Geometry: final body of the model. Coordinates: model frame, mm. Face numbers are marked on the shaded views. A direction names the side the tool comes from. Give positions to 0.01 mm unless a question says otherwise; leave off trailing zeros. Write each loop counter-clockwise with the first axis right and the second up, starting at its lowest first coordinate (ties: lowest second). Pieces come first, ordered by that corner, then holes. Notation, with made-up numbers: (12.25, 44) - (53.25, 44) arc R14 ccw to (53.25, 54) - close; hole circle Ø6 at (-28.5, -35.5). An arc over 180 degrees is marked (long way). One line per question, with ' | ' between items. Start each with the question number.
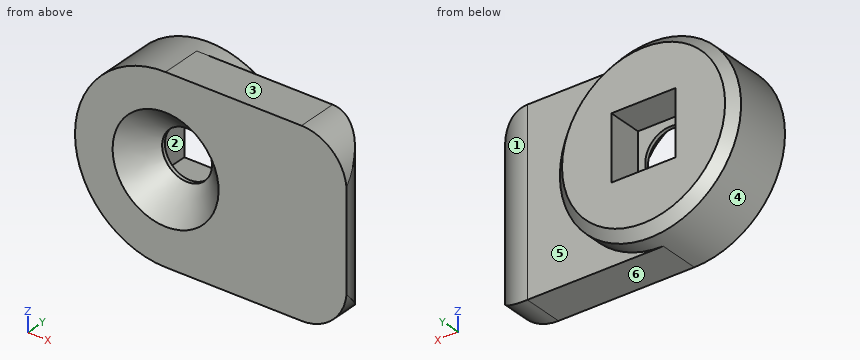
Autodesk Inventor part; units mm, degrees
ref_plane "bottom_to_ins_XY" through (0, 0, 0) normal (0, 1, 0) x (1, 0, 0)
ref_plane "bottom_to_ins_YZ" through (0, 0, 0) normal (1, 0, 0) x (0, 0, -1)
ref_plane "bottom_to_ins_ZX" through (0, 0, 0) normal (0, 0, -1) x (0, 1, 0)
sketch "Sketch_1" plane through (0, 0, 0) normal (0, 0, 1) x (1, 0, 0)
  line L0 (0, -10) -> (0, -2.65)
  line L1 (0, -2.65) -> (9, -2.65)
  line L2 (9, -2.65) -> (10, -3.65)
  line L3 (10, -3.65) -> (10, -10)
  line L4 (10, -10) -> (0, -10)
  line L5 (0, -10) -> (0, -2.65)
revolve "Revolution1" add sketch "Sketch_1" angle 360 about axis through (0, -10, 0) along (0, -1, 0)
sketch "Sketch_2" plane through (0, -10, 0) normal (0, 1, 0) x (1, 0, 0)
  line L0 (0, 10) -> (0, -10)
  line L1 (0, -10) -> (15, -10)
  arc A0 (15, -10) -> (20, -5) centre (15, -5) ccw
  line L2 (20, -5) -> (20, 5)
  arc A1 (20, 5) -> (15, 10) centre (15, 5) ccw
  line L3 (15, 10) -> (0, 10)
extrude "Extrusion1" add sketch "Sketch_2" along normal blind 4.5
sketch "Sketch3" plane through (0, -10, -10) normal (0, -1, 0) x (1, 0, 0)
  point P0 (0, 10)
hole "Hole1" at (0, -10, 0) direction (0, 1, 0) diameter 5.5 depth 3.5 countersink diameter 11.7 countersink angle 90
sketch "Sketch_9" plane through (0, 0, 0) normal (0, 1, 0) x (-1, 0, 0)
  line L0 (3.55, -3.55) -> (3.55, 3.55)
  line L1 (3.55, 3.55) -> (-3.55, 3.55)
  line L2 (-3.55, 3.55) -> (-3.55, -3.55)
  line L3 (-3.55, -3.55) -> (3.55, -3.55)
extrude "Extrusion2" cut sketch "Sketch_9" against normal blind 6.5
sketch "Sketch_3" plane through (0, 0, 0) normal (0, 0, 1) x (1, 0, 0)
  line L0 (15, -2) -> (15, -5.5)
  arc A0 (20, -10.5) -> (15, -5.5) centre (15, -10.5) ccw
  line L1 (20, -10.5) -> (25, -10.5)
  line L2 (25, -10.5) -> (25, -2)
  line L3 (25, -2) -> (15, -2)
extrude "Extrusion3" cut sketch "Sketch_3" along normal mid plane 20
ref_plane "bottom_to_ins_XY" through (0, 0, 0) normal (0, 1, 0) x (1, 0, 0)
ref_plane "bottom_to_ins_YZ" through (0, 0, 0) normal (1, 0, 0) x (0, 0, -1)
ref_plane "bottom_to_ins_ZX" through (0, 0, 0) normal (0, 0, -1) x (0, 1, 0)
properties part number "JBlock_plate"
1) Section A-A, the plane y = -7.5. Output: boundary loops of the cut face in (x, z).
2) Reachability of the marked faces 4, 5 and 6 from +Z, -Z, +X, -X, +Y, -Y: full face, straight path, thin tool, end or side. Return the list, or none.
3) Section B-B, the plane z = 0. Output: boundary loops of the cut face in (x, y), plus the area to 3 significant figures.
4) Section D-D, the plane x = 17.5. Output: boundary loops of the cut face in (y, z).
5) Section C-C, the plane y = -3.25. Output: boundary loops of the cut face in (x, z), plus the area to 3 significant figures.
6) Pull-direction query (X, two-part tool) for the marked faces 1, 2 and 3; classes: +X half, -X half, draft (parallel to the pull), parting line (faces both ways), or undercut.
7) First-contact query: pin 1 Ø1 at (x, y) = (-1.5, -5) entering from +Z; pin 2 Ø3.5 at (x, z) = (0, -0.5) entering from +Y; pin 3 Ø1 at (y, z) = (-9, -7) entering from +X; pin 4 Ø3 at (x, y) = (6, -3.5) entering from +Z. Flat tips, straight axial feed; report the tip coordinate or a pass-through.
8) Line query: L1, parallel to Z at x = 2.5, y = -8.5; L2, parallel to Z at x = 0, y = -6.8; L3, parallel to Y at x = 10.75, z = 8. Output: solid intervals per line, ascending.
Answer key:
1) outline: (0, -10) - (15, -10) arc R5 ccw to (19, -8) - (19, 8) arc R5 ccw to (15, 10) - (0, 10) arc R10 ccw to start; hole circle Ø6.7 at (0, 0)
2) face 4: +Y | face 5: +X, +Y | face 6: -Z, +X, -X, +Y, -Y
3) outline: (-10, -10) - (-5.85, -10) - (-2.75, -6.9) - (-2.75, -6.5) - (-3.55, -6.5) - (-3.55, -2.65) - (-9, -2.65) - (-10, -3.65) - close; (2.75, -6.9) - (5.85, -10) - (19.97, -10) arc R5 ccw to (15, -5.5) - (10, -5.5) - (10, -3.65) - (9, -2.65) - (3.55, -2.65) - (3.55, -6.5) - (2.75, -6.5) - close | area: 129 mm^2
4) outline: (-10, -9.33) - (-6.17, -9.33) - (-6.17, 9.33) - (-10, 9.33) - close
5) outline: circle Ø19.2 at (0, 0); hole (-3.55, -3.55) - (3.55, -3.55) - (3.55, 3.55) - (-3.55, 3.55) - close | area: 239 mm^2
6) face 1: +X half | face 2: undercut | face 3: draft
7) pin 1: z = 9.95 | pin 2: through | pin 3: x = 19.77 | pin 4: z = 8.93
8) L1: -10 to -3.56, 3.56 to 10 | L2: -10 to -2.75, 2.75 to 10 | L3: -10 to -5.5
